```python
from build123d import *

# Parameters (mm, degrees)
SKETCH1_R           = 10.16
BOSS_EXTRUDE1_DEPTH = 28
SKETCH2_R           = 12.7
BOSS_EXTRUDE2_DEPTH = 5.08
BOSS_EXTRUDE3_DEPTH = 5.715
FILLET1_R           = 1.27
FILLET2_R           = 0.508


with BuildPart() as part:
    # Sketch1 → Boss-Extrude1 (new body)
    with BuildSketch(Plane.XY):
        Circle(SKETCH1_R)
    extrude(amount=BOSS_EXTRUDE1_DEPTH)

    # Sketch2 → Boss-Extrude2 (add)
    with BuildSketch(Plane.XY.offset(28)):
        Circle(SKETCH2_R)
    extrude(amount=BOSS_EXTRUDE2_DEPTH)

    # Sketch3 → Boss-Extrude3 (add, symmetric)
    with BuildSketch(Plane(origin=(0, 0, 0), x_dir=(0, 0, -1), z_dir=(1, 0, 0))):
        with BuildLine():
            Line((-33.08, -8.833721506), (-33.08, 10.59406456))
            Line((-33.08, 10.59406456), (-37.824147833, 10.59406456))
            add(Edge.make_bspline(
                [(-37.824147833, 10.59406456), (-35.198663917, 1.074784021), (-35.199636371, -8.833721506)],
                knots=[0, 0, 0, 1, 1, 1], degree=2))
            Line((-35.199636371, -8.833721506), (-33.08, -8.833721506))
        make_face()
    extrude(amount=BOSS_EXTRUDE3_DEPTH, both=True)

    # Fillet1
    fillet1_edges = [part.edges().sort_by_distance(p)[0] for p in [
        (-2.8575, -8.833721506, 35.199636371),
        (-5.715, 0.969066451, 35.854142221),
        (-2.8575, 10.59406456, 37.824147833),
        (5.715, 0.969066451, 35.854142221),
    ]]
    fillet(fillet1_edges, radius=FILLET1_R)

    # Fillet2
    fillet2_edges = [part.edges().sort_by_distance(p)[0] for p in [
        (-12.7, 0, 33.08),
    ]]
    fillet(fillet2_edges, radius=FILLET2_R)


solid = part.part
```
The model under review builds one solid part; all positions refer to its coordinate system, in mm. A direction names the side the tool comes from. Round coordinates to 2 decimals unless told otherwise and drop trailing zeros. Loops run counter-clockwise (first coordinate to the right, second up) from the corner with the lowest first, then second, coordinate; pieces in that order, holes last. Notation, with made-up numbers: (50, 1.5) - (81, 1.5) arc R20 ccw to (81, 21.5) - close; hole circle Ø7 at (64, -15). An arc over 180 degrees is marked (long way). Use a Markdown table: item, result. Add a question column.
Q1. Add section A-A (z = 6.5). State the section outline as (x, y) points.
Q2. Add section B-B (z = 33.5). State the section outline as (x, y) points (3 decimals).
Q3. For probe 1 along Z at (x, y) = (10.5, 0); probe 2 along X at (y, z) = (10, 36.5); probe 3 along Z at (x, y) = (8.75, 0), list the stretches that pass through material, from the lowest coordinate up.
Q4. Insertion check: pin 1 Ø2.5 at (y, z) = (4.5, 34.5) entering from -X (3 decimals); pin 2 Ø0.7 at (x, z) = (-1.5, 33.5) entering from -Y; pin 3 Ø1.5 at (x, z) = (-1.5, 12.5) entering from -Y. Each pin has a flat end and moves straight along its axis. Give the tip position at first contact, or say it passes through.
Q5. Machinability: for faces 1 (the face through (0, 10.594, 35)), 2 (the face through (0.1, -8.834, 33.5)), 3 (the face through (-6, 9, 28)), 4 (the face through (-5.715, 3, 34)), which of the approach directions +Z, -Z, +X, -X, +Y, -Y give a long, thin tool a straight path to every point of the face, cutting with its end or side? Answer none if there is none.
Worked answers:
| question | item | result |
|---|---|---|
| 1 | outline | circle Ø20.32 at (0, 0) |
| 2 | outline | (-5.715, -8.834) - (5.715, -8.834) - (5.715, 10.594) - (-5.715, 10.594) - close |
| 3 | probe 1 | 28 to 33.08 |
| 3 | probe 2 | -5.71 to 5.71 |
| 3 | probe 3 | 0 to 33.08 |
| 4 | pin 1 | x = -5.715 |
| 4 | pin 2 | y = -8.83 |
| 4 | pin 3 | y = -10.13 |
| 5 | face 1 | +Z, +X, -X, +Y |
| 5 | face 2 | +Z, +X, -X, -Y |
| 5 | face 3 | -Z |
| 5 | face 4 | +Z, -X, +Y, -Y |
